```python
from build123d import *

# Parameters (mm, degrees)
F0_W     = 45.72
F0_H     = 25.4
F0_W_2   = 19.05
F0_H_2   = 5.1054
F1_DEPTH = 12.7
F3_D     = 6.477


with BuildPart() as f1:
    # F0 (on Top) → F1 (new body)
    with BuildSketch(Plane.XY):
        Rectangle(F0_W, F0_H)
        Rectangle(F0_W_2, F0_H_2, mode=Mode.SUBTRACT)
    extrude(amount=F1_DEPTH)

    # F3 (through all)
    with Locations(Plane.XZ.offset(12.7)):
        with Locations((-19.446875, 6.35), (19.446875, 6.35)):
            Hole(F3_D / 2)


solid = f1.part
```
Work out the finished part from the listing and answer in its coordinate system (mm). A direction names the side the tool comes from. Give positions to 0.01 mm unless a question says otherwise; leave off trailing zeros. Loops run counter-clockwise (first coordinate to the right, second up) from the corner with the lowest first, then second, coordinate; pieces in that order, holes last. Notation, with made-up numbers: (75, -31.5) -> (98, -31.5) arc R13 ccw to (98, -21.5) -> close; hole circle Ø8 at (61, 52). An arc over 180 degrees is marked (long way). Write item = value, one per line. Start each with the question number.
(1) Find section B-B on y = -0.75. Give the number of separate pieces and of enclosed holes in the cut face, and give its area (3 significant figures).
(2) Find section C-C on z = 1.25. Give the vertices of the cut face in (x, y) (3 decimals).
(3) Given pin 1 Ø7.5 at (x, z) = (19.45, 6.35) entering from -Y; pin 2 Ø6 at (x, z) = (-19.45, 6.35) entering from +Y, each flat-ended and moving along its own axis, determine where each tip first touches the part or whether it passes through.
(4) Which of the six approach directions +Z, -Z, +X, -X, +Y, -Y give full straight-line access (tool end or side, diameter ignored) to faces 4 (the flat face through (9.525, 0, 6)), 5 (the flat face through (22.86, 0, 6))?
(5) Find section A-A on z = 6.35. Give the vertices of the cut face in (x, y) (3 decimals).
(6) The mould has two halves that part along Y. Classify faces 1 (the flat face through (0, 2.553, 6)), 2 (the flat face through (0, 12.7, 6)), 3 (the cylindrical face through (22.682, 0.178, 6.492)): +Y half, -Y half, draft (parallel to the pull), parting line (faces both ways), or undercut.
(7) Find section D-D on y = 6.25. Give the vertices of the cut face in (x, z).
(8) Find the intervals of material crossed by probe 1 along Y at (x, z) = (8.5, 3.5); probe 2 along X at (y, z) = (-0.5, 6.5) (3 decimals); probe 3 along X at (y, z) = (0.5, 8.5) (3 decimals), in increasing order. Write a range as from..to.
From the geometry:
q1.separate_pieces = 2
q1.enclosed_holes = 2
q1.area = 273 mm^2
q2.outline = (-22.86, -12.7) -> (22.86, -12.7) -> (22.86, 12.7) -> (-22.86, 12.7) -> close; hole (-9.525, -2.553) -> (9.525, -2.553) -> (9.525, 2.553) -> (-9.525, 2.553) -> close
q3.pin_1 = -12.7
q3.pin_2 = through
q4.face_4 = +Z, -Z
q4.face_5 = +Z, -Z, +X, +Y, -Y
q5.outline = (-22.86, -12.7) -> (-22.685, -12.7) -> (-22.685, 12.7) -> (-22.86, 12.7) -> close; (-16.208, -12.7) -> (16.208, -12.7) -> (16.208, 12.7) -> (-16.208, 12.7) -> close; (22.685, -12.7) -> (22.86, -12.7) -> (22.86, 12.7) -> (22.685, 12.7) -> close; hole (-9.525, -2.553) -> (9.525, -2.553) -> (9.525, 2.553) -> (-9.525, 2.553) -> close
q6.face_1 = undercut
q6.face_2 = +Y half
q6.face_3 = draft
q7.outline = (-22.86, 0) -> (22.86, 0) -> (22.86, 12.7) -> (-22.86, 12.7) -> close; hole circle Ø6.48 at (-19.45, 6.35); hole circle Ø6.48 at (19.45, 6.35)
q8.probe_1 = -12.7..-2.55, 2.55..12.7
q8.probe_2 = -22.86..-22.682, -16.212..-9.525, 9.525..16.212, 22.682..22.86
q8.probe_3 = -22.86..-21.869, -17.025..-9.525, 9.525..17.025, 21.869..22.86
